Verification items for the finished model (mm, model axes). A direction names the side the tool comes from. Coordinates: 2 decimals unless noted, no trailing zeros. Write each loop counter-clockwise with the first axis right and the second up, starting at its lowest first coordinate (ties: lowest second). Pieces come first, ordered by that corner, then holes. Notation, with made-up numbers: (71, 58) -> (79, 58) arc R9 ccw to (79, 64) -> close; hole circle Ø9 at (-0.5, 88). An arc over 180 degrees is marked (long way). Answer in a Markdown table with one row per item.
```python
from build123d import *

# Parameters (mm, degrees)
EXTRUDE_1_DEPTH     = 46
CUT_EXTRUDE_1_DEPTH = 3
SKETCH_3_R          = 1.75
CUT_EXTRUDE_2_DEPTH = 26.47


with BuildPart() as part:
    # Эскиз1 → Бобышка-Вытянуть1 (new body)
    with BuildSketch(Plane(origin=(0, 0, 0), x_dir=(1, 0, 0), z_dir=(0, 1, 0))):
        with BuildLine():
            Line((-14.235, 20), (14.235, 20))
            Line((14.235, 20), (14.235, -20))
            Line((14.235, -20), (1.903095238, -20))
            Line((1.903095238, -20), (1.903095238, -5.624459703))
            ThreePointArc((1.903095238, -5.624459703), (0.265, 15.75), (-1.373095238, -5.624459703))
            Line((-1.373095238, -5.624459703), (-1.373095238, -20))
            Line((-1.373095238, -20), (-14.235, -20))
            Line((-14.235, -20), (-14.235, 20))
        make_face()
    extrude(amount=EXTRUDE_1_DEPTH)

    # Эскиз2 → Вырез-Вытянуть1 (cut)
    with BuildSketch(Plane.ZY.offset(14.235)):
        Polygon((12.733013434, 19.75), (15.547595996, 21.375), (15.547595996, 24.625), (12.733013434, 26.25), (9.918430872, 24.625), (9.918430872, 21.375), align=None)
    extrude(amount=-CUT_EXTRUDE_1_DEPTH, mode=Mode.SUBTRACT)

    # Эскиз3 → Вырез-Вытянуть2 (cut, through all)
    with BuildSketch(Plane.ZY.offset(11.235)):
        with Locations((12.733013434, 23)):
            Circle(SKETCH_3_R)
    extrude(amount=-CUT_EXTRUDE_2_DEPTH, mode=Mode.SUBTRACT)


solid = part.part
```
1. Depth check by flat-ended pin: P1, Ø5, axis at x = 1, y = 19, coming from the +Z side; P2, Ø5.5, axis at y = 23, z = 12.73, coming from the -X side (3 decimals). Enter the tip coordinate at first touch or a pass-through.
Geometry says:
| item | result |
|---|---|
| P1 | z = 20 |
| P2 | x = -11.235 |
2. Section check C-C, the plane x = 3.25. Record the boundary of the cut face in (y, z).
Geometry says:
| item | result |
|---|---|
| outline | (0, -20) -> (46, -20) -> (46, -15.33) -> (0, -15.33) -> close; (0, 5.33) -> (46, 5.33) -> (46, 20) -> (0, 20) -> close; hole circle Ø3.5 at (23, 12.73) |
3. Section check B-B, the plane y = 23. Record the boundary of the cut face in (x, z) (3 decimals).
Geometry says:
| item | result |
|---|---|
| outline | (-14.235, -20) -> (14.235, -20) -> (14.235, 10.983) -> (1.903, 10.983) -> (1.903, 5.624) arc R10.75 cw (long way) to (-1.373, 5.624) -> (-1.373, 10.983) -> (-11.235, 10.983) -> (-11.235, 9.918) -> (-14.235, 9.918) -> close; (-14.235, 15.548) -> (-11.235, 15.548) -> (-11.235, 14.483) -> (-1.373, 14.483) -> (-1.373, 20) -> (-14.235, 20) -> close; (1.903, 14.483) -> (14.235, 14.483) -> (14.235, 20) -> (1.903, 20) -> close |
4. Thickness scan on line 1 (X direction, y = 8, z = 16) (3 decimals); line 2 (X direction, y = 30, z = -5) (3 decimals); line 3 (Z direction, x = 5.25, y = 22). Record the ranges inside material, lowest first. Write a range as from..to.
Geometry says:
| item | result |
|---|---|
| line 1 | -14.235..-1.373, 1.903..14.235 |
| line 2 | -14.235..-10.485, 11.015..14.235 |
| line 3 | -20..-14.52, 4.52..11.3, 14.17..20 |
5. Mould release check, pull along X, two halves, no side actions. Record for faces 1 (the flat face through (-11.235, 22, 11)), 2 (the flat face through (-1.373, 23, 10)), 3 (the flat face through (-13, 23, 15.548)): released by +X, released by -X, zero draft, split by the parting line, or undercut.
Geometry says:
| item | result |
|---|---|
| face 1 | released by -X |
| face 2 | undercut |
| face 3 | zero draft |
6. Section check A-A, the plane z = -5. Record the boundary of the cut face in (x, y) (3 decimals).
Geometry says:
| item | result |
|---|---|
| outline | (-14.235, 0) -> (-10.485, 0) -> (-10.485, 46) -> (-14.235, 46) -> close; (11.015, 0) -> (14.235, 0) -> (14.235, 46) -> (11.015, 46) -> close |
7. Section check D-D, the plane y = 15.5. Record the boundary of the cut face in (x, z) (3 decimals), plus the area to 3 significant figures.
Geometry says:
| item | result |
|---|---|
| outline | (-14.235, -20) -> (14.235, -20) -> (14.235, 20) -> (1.903, 20) -> (1.903, 5.624) arc R10.75 cw (long way) to (-1.373, 5.624) -> (-1.373, 20) -> (-14.235, 20) -> close |
| area | 729 mm^2 |
8. Tool access check on faces 4 (the flat face through (-12.76, 25.45, 11.35)), 5 (the flat face through (8, 23, 20)), 6 (the flat face through (1.903, 23, 15)). Record the directions out of +Z, -Z, +X, -X, +Y, -Y that give a thin tool (end or side, any length) a straight path to the whole face; none if there is none.
Geometry says:
| item | result |
|---|---|
| face 4 | -X |
| face 5 | +Z, +X, -X, +Y, -Y |
| face 6 | +Z, +Y, -Y |
